```python
from build123d import *

# Parameters (mm, degrees)
SKETCH1_W           = 35
SKETCH1_H           = 36.5
BOSS_EXTRUDE1_DEPTH = 2.5
SKETCH3_R           = 3.5
CUT_EXTRUDE1_DEPTH  = 35
SKETCH4_R           = 2.5
BOSS_EXTRUDE3_DEPTH = 4
SKETCH5_W           = 1.5
SKETCH5_H           = 3
BOSS_EXTRUDE4_DEPTH = 5
CUT_EXTRUDE2_REACH  = 55.456
SKETCH6_R           = 1
FILLET1_R           = 1
FILLET2_R           = 1
SKETCH7_R           = 6
CUT_EXTRUDE3_DEPTH  = 5
FILLET3_R           = 2


with BuildPart() as part:
    # Sketch1 → Boss-Extrude1 (new, symmetric)
    with BuildSketch(Plane.XY):
        with Locations((17.5, 18.25)):
            Rectangle(SKETCH1_W, SKETCH1_H)
    extrude(amount=BOSS_EXTRUDE1_DEPTH, both=True)

    # Sketch3 → Cut-Extrude1 (cut)
    with BuildSketch(Plane(origin=(35, 0, 0), x_dir=(0, 0, -1), z_dir=(1, 0, 0))):
        with Locations((1, 0)):
            Circle(SKETCH3_R)
    extrude(amount=-CUT_EXTRUDE1_DEPTH, mode=Mode.SUBTRACT)

    # Sketch4 → Boss-Extrude3 (add)
    # profile 1 of 2: a face of its own
    with BuildSketch(Plane(origin=(35, 0, 0), x_dir=(0, 0, -1), z_dir=(1, 0, 0))):
        with BuildLine():
            ThreePointArc((2.5, 3.16227766), (-0.870828693, 2.958039892), (-2.5, 0))
            ThreePointArc((-2.5, 0), (-1.474873734, -2.474873734), (1, -3.5))
            ThreePointArc((1, -3.5), (3.474873734, -2.474873734), (4.5, 0))
            ThreePointArc((4.5, 0), (3.958039892, 1.870828693), (2.5, 3.16227766))
        make_face()
        with Locations((1, 0)):
            Circle(SKETCH4_R, mode=Mode.SUBTRACT)
    # profile 2 of 2: a face of its own
    with BuildSketch(Plane(origin=(35, 0, 0), x_dir=(0, 0, -1), z_dir=(1, 0, 0))):
        with BuildLine():
            ThreePointArc((1, -3.5), (-1.474873734, -2.474873734), (-2.5, 0))
            Line((-2.5, 0), (-2.5, -3.5))
            Line((-2.5, -3.5), (1, -3.5))
        make_face()
    boss_extrude3 = extrude(amount=-BOSS_EXTRUDE3_DEPTH)

    # Mirror2: Boss-Extrude3 across plane
    add(boss_extrude3.mirror(Plane(origin=(17.5, 0, 0), x_dir=(0, 0, 1), z_dir=(1, 0, 0))))

    # Sketch5 → Boss-Extrude4 (add, symmetric)
    with BuildSketch(Plane(origin=(17.5, 0, 0), x_dir=(0, 0, -1), z_dir=(1, 0, 0))):
        with Locations((-3.25, 38)):
            Rectangle(SKETCH5_W, SKETCH5_H)
        Polygon((-4, 36.5), (-2.5, 35), (-2.5, 36.5), align=None)
        Polygon((2.5, 35), (2.5, 36.5), (4, 36.5), align=None)
        with Locations((3.25, 38)):
            Rectangle(SKETCH5_W, SKETCH5_H)
    extrude(amount=BOSS_EXTRUDE4_DEPTH, both=True)

    # Cut-Extrude2: up to this face of the body (flat: up to its plane)
    cut_extrude2_end = Plane(part.part.faces().sort_by_distance((17.5, 38, -4))[0])
    # Sketch6 → Cut-Extrude2 (cut, up to the picked face)
    with BuildSketch(Plane.XY.offset(4), mode=Mode.PRIVATE) as cut_extrude2_sk1:
        with Locations(Location((17.5, 38, 0), (0, 0, 270))):
            Circle(SKETCH6_R)
    cut_extrude2_tool1 = split(extrude(cut_extrude2_sk1.sketch, amount=-CUT_EXTRUDE2_REACH, mode=Mode.PRIVATE), bisect_by=cut_extrude2_end, keep=Keep.BOTH, mode=Mode.PRIVATE)
    add(cut_extrude2_tool1.solids().sort_by(Axis((17.5, 38, 4), (0, 0, -1)))[0], mode=Mode.SUBTRACT)

    # Fillet1
    fillet1_edges = [part.edges().sort_by_distance(p)[0] for p in [
        (12.5, 35.75, 3.25),
        (17.5, 36.5, 4),
        (22.5, 35.75, 3.25),
        (22.5, 35.75, -3.25),
        (17.5, 36.5, -4),
        (12.5, 35.75, -3.25),
    ]]
    fillet(fillet1_edges, radius=FILLET1_R)

    # Fillet2
    fillet2_edges = [part.edges().sort_by_distance(p)[0] for p in [
        (22.5, 39.5, 3.25),
        (12.5, 39.5, 3.25),
        (22.5, 39.5, -3.25),
        (12.5, 39.5, -3.25),
    ]]
    fillet(fillet2_edges, radius=FILLET2_R)

    # Sketch7 → Cut-Extrude3 (cut)
    with BuildSketch(Plane.XY.offset(2.5)):
        with Locations((0, 36.5)):
            Circle(SKETCH7_R)
    extrude(amount=-CUT_EXTRUDE3_DEPTH, mode=Mode.SUBTRACT)

    # Fillet3
    # the kernel refuses this fillet: 2 mm, written as the material it takes off along each edge
    with BuildSketch(Plane(origin=(35, -8.5, 2.5), x_dir=(-1, 0, 0), z_dir=(0, 1, 0))) as fillet3_piece_1:
        with BuildLine():
            CenterArc((FILLET3_R, -FILLET3_R), FILLET3_R, 90, 90)
            Line((0, -FILLET3_R), (0, 0))
            Line((0, 0), (FILLET3_R, 0))
        make_face()
    extrude(amount=50, mode=Mode.SUBTRACT)


solid = part.part
```
Input: part model. Units: mm. Frame: model coordinates. Round coordinates to 2 decimals unless told otherwise and drop trailing zeros. Loops run counter-clockwise (first coordinate to the right, second up) from the corner with the lowest first, then second, coordinate; pieces in that order, holes last. Notation, with made-up numbers: (-32.75, -7.5) - (4.25, -7.5) arc R26 cw to (4.25, 10.5) - close; hole circle Ø9 at (10.25, 42). An arc over 180 degrees is marked (long way). One line per item, written item: value. Start each with the question number.
(1) Ray query, line 1 (Z direction, x = 18.5, y = 17.5); line 2 (Y direction, x = 32.3, z = -1); line 3 (Y direction, x = 0.95, z = -1). Return the intervals inside material, ascending. Write a range as [from, to].
(2) Section C-C, the plane x = 26.5. Return loops of the section in (y, z).
(3) Section B-B, the plane x = 3.5. Return loops of the section in (y, z).
(4) Draft query along X for faces 1 (the flat face through (4, -2, 1)), 2 (the cylindrical face through (4.196, 32.211, 0.035)), 3 (the flat face through (17, 39.5, 3)). Return one class per face: +X half, -X half, draft (parallel to the pull), parting line (faces both ways), or undercut.
(5) Section A-A, the plane y = 12. Return loops of the section in (x, z), plus the area to 3 significant figures.
(6) Contact query for flat-ended pins moving along their axis: P1, Ø1.5, axis at x = 13.5, z = 0.5, coming from the -Y side; P2, Ø16.5, axis at x = 8.5, y = 10, coming from the +Z side; P3, Ø0.8, axis at y = 37.5, z = -3, coming from the +X side. Output: stop coordinate, or through.
(7) Section D-D, the plane y = 31.5. Return loops of the section in (x, z), plus the area to 3 significant figures.
Results below:
1. line 1: [-2.5, 2.5]
1. line 2: [-3.5, -2.5], [2.5, 36.5]
1. line 3: [-3.5, -2.5], [2.5, 30.58]
2. outline: (0, 2.5) arc R3.5 cw to (3.16, -2.5) - (36.5, -2.5) - (36.5, 2.5) - close
3. outline: (-3.5, -1) arc R3.5 ccw to (3.16, -2.5) - (31.63, -2.5) - (31.63, 2.5) - (-3.5, 2.5) - close; hole circle Ø5 at (0, -1)
4. face 1: undercut
4. face 2: -X half
4. face 3: draft
5. outline: (0, -2.5) - (35, -2.5) - (35, 0.5) arc R2 ccw to (33, 2.5) - (0, 2.5) - close
5. area: 174 mm^2
6. P1: y = 2.68
6. P2: z = 2.5
6. P3: x = 22.5
7. outline: (3.32, -2.5) - (35, -2.5) - (35, 0.5) arc R2 ccw to (33, 2.5) - (3.32, 2.5) - close
7. area: 158 mm^2
